```python
from build123d import *

# Parameters (mm, degrees)
SKETCH1_W           = 45
SKETCH1_H           = 30
BOSS_EXTRUDE1_DEPTH = 5
CUT_EXTRUDE1_REACH  = 7
SKETCH2_R           = 1.6
SKETCH4_W           = 45
SKETCH4_H           = 5
BOSS_EXTRUDE2_DEPTH = 55
SKETCH5_W           = 45
SKETCH5_H           = 5
BOSS_EXTRUDE3_DEPTH = 75


with BuildPart() as part:
    # Sketch1 → Boss-Extrude1 (new body)
    with BuildSketch(Plane(origin=(0, 0, 0), x_dir=(1, 0, 0), z_dir=(0, 1, 0))):
        Rectangle(SKETCH1_W, SKETCH1_H)
    extrude(amount=BOSS_EXTRUDE1_DEPTH)

    # Sketch2 → Cut-Extrude1 (cut, up to next)
    with BuildSketch(Plane(origin=(0, 0, 0), x_dir=(1, 0, 0), z_dir=(0, 1, 0)), mode=Mode.PRIVATE) as cut_extrude1_sk1:
        with Locations((-15, 7.5)):
            Circle(SKETCH2_R)
    cut_extrude1_tool1 = extrude(cut_extrude1_sk1.sketch, amount=CUT_EXTRUDE1_REACH, mode=Mode.PRIVATE) & part.part
    add(cut_extrude1_tool1.solids().sort_by_distance((-15, 0, -7.5))[0], mode=Mode.SUBTRACT)
    # Sketch2 → Cut-Extrude1 (cut, up to next)
    with BuildSketch(Plane(origin=(0, 0, 0), x_dir=(1, 0, 0), z_dir=(0, 1, 0)), mode=Mode.PRIVATE) as cut_extrude1_sk2:
        with Locations((15, 7.5)):
            Circle(SKETCH2_R)
    cut_extrude1_tool2 = extrude(cut_extrude1_sk2.sketch, amount=CUT_EXTRUDE1_REACH, mode=Mode.PRIVATE) & part.part
    add(cut_extrude1_tool2.solids().sort_by_distance((15, 0, -7.5))[0], mode=Mode.SUBTRACT)
    # Sketch2 → Cut-Extrude1 (cut, up to next)
    with BuildSketch(Plane(origin=(0, 0, 0), x_dir=(1, 0, 0), z_dir=(0, 1, 0)), mode=Mode.PRIVATE) as cut_extrude1_sk3:
        with Locations((15, -7.5)):
            Circle(SKETCH2_R)
    cut_extrude1_tool3 = extrude(cut_extrude1_sk3.sketch, amount=CUT_EXTRUDE1_REACH, mode=Mode.PRIVATE) & part.part
    add(cut_extrude1_tool3.solids().sort_by_distance((15, 0, 7.5))[0], mode=Mode.SUBTRACT)
    # Sketch2 → Cut-Extrude1 (cut, up to next)
    with BuildSketch(Plane(origin=(0, 0, 0), x_dir=(1, 0, 0), z_dir=(0, 1, 0)), mode=Mode.PRIVATE) as cut_extrude1_sk4:
        with Locations((-15, -7.5)):
            Circle(SKETCH2_R)
    cut_extrude1_tool4 = extrude(cut_extrude1_sk4.sketch, amount=CUT_EXTRUDE1_REACH, mode=Mode.PRIVATE) & part.part
    add(cut_extrude1_tool4.solids().sort_by_distance((-15, 0, 7.5))[0], mode=Mode.SUBTRACT)

    # Sketch4 → Boss-Extrude2 (add)
    with BuildSketch(Plane.XY.offset(15)):
        with Locations((0, 2.5)):
            Rectangle(SKETCH4_W, SKETCH4_H)
    extrude(amount=BOSS_EXTRUDE2_DEPTH)

    # Sketch5 → Boss-Extrude3 (add)
    with BuildSketch(Plane(origin=(0, 5, 0), x_dir=(1, 0, 0), z_dir=(0, 1, 0))):
        with Locations((0, -67.5)):
            Rectangle(SKETCH5_W, SKETCH5_H)
    extrude(amount=BOSS_EXTRUDE3_DEPTH)


solid = part.part
```
Verification items for the finished model (mm, model axes). A direction names the side the tool comes from. Give positions to 0.01 mm unless a question says otherwise; leave off trailing zeros. Loops run counter-clockwise (first coordinate to the right, second up) from the corner with the lowest first, then second, coordinate; pieces in that order, holes last. Notation, with made-up numbers: M 12.5,67.5 L 62.5,67.5 A15 cw 62.5,75.5 Z; hole C 23,73.25 d4. An arc over 180 degrees is marked long. Return JSON: item names as keys, results as strings.
1) Section check B-B, the plane z = 7.5. Enter the section's corners in (x, y), and give its area (3 significant figures).
Findings:
{"outline": "M -22.5,0 L -16.6,0 L -16.6,5 L -22.5,5 Z; M -13.4,0 L 13.4,0 L 13.4,5 L -13.4,5 Z; M 16.6,0 L 22.5,0 L 22.5,5 L 16.6,5 Z", "area": "193 mm2"}
2) Tool access check on faces 5 (the cylindrical face through (-16.27, 2.46, 8.47)), 6 (the flat face through (0, 42, 65)). Record the directions out of +Z, -Z, +X, -X, +Y, -Y that give a thin tool (end or side, any length) a straight path to the whole face; none if there is none.
Findings:
{"face 5": "+Y, -Y", "face 6": "-Z, +X, -X, +Y"}
3) Gauge pin test, flat ends, axial feed: P1, Ø6, axis at x = -10, z = 21, coming from the +Y side; P2, Ø1.9, axis at x = 15, z = 7.5, coming from the -Y side; P3, Ø2, axis at x = -12, y = 19.5, coming from the -Z side. Record the tip position at first contact, or that the pin passes through.
Findings:
{"P1": "stops at y = 5", "P2": "passes through", "P3": "stops at z = 65"}
4) Material ranges on L1, parallel to Z at x = 15, y = 1; L2, parallel to X at y = 3.8, z = -7.5; L3, parallel to X at y = 3, z = 7, recorded low to high. Write a range as [from, to].
Findings:
{"L1": "z = [-15, -9.1], [-5.9, 5.9], [9.1, 70]", "L2": "x = [-22.5, -16.6], [-13.4, 13.4], [16.6, 22.5]", "L3": "x = [-22.5, -16.52], [-13.48, 13.48], [16.52, 22.5]"}
5) Mould release check, pull along X, two halves, no side actions. Record for faces 1 (the flat face through (22.5, 4, 47)), 2 (the flat face through (0, 39, 70)), 3 (the flat face through (-22.5, 4, 47)), 4 (the cylindrical face through (13.4, 2.46, -7.57)): released by +X, released by -X, zero draft, split by the parting line, or undercut.
Findings:
{"face 1": "released by +X", "face 2": "zero draft", "face 3": "released by -X", "face 4": "undercut"}
6) Section check A-A, the plane x = -15. Enter the section's corners in (y, z), and give its area (3 significant figures).
Findings:
{"outline": "M 0,-15 L 5,-15 L 5,-9.1 L 0,-9.1 Z; M 0,-5.9 L 5,-5.9 L 5,5.9 L 0,5.9 Z; M 0,9.1 L 5,9.1 L 5,65 L 80,65 L 80,70 L 0,70 Z", "area": "768 mm2"}
7) Section check D-D, the plane z = 25. Enter the section's corners in (x, y).
Findings:
{"outline": "M -22.5,0 L 22.5,0 L 22.5,5 L -22.5,5 Z"}
8) Section check C-C, the plane x = 2. Enter the section's corners in (y, z).
Findings:
{"outline": "M 0,-15 L 5,-15 L 5,65 L 80,65 L 80,70 L 0,70 Z"}
